Source: CAD feature listing. Evaluate the final solid. Frame: model axes, mm. A direction names the side the tool comes from. Round coordinates to 2 decimals unless told otherwise and drop trailing zeros. Loops run counter-clockwise (first coordinate to the right, second up) from the corner with the lowest first, then second, coordinate; pieces in that order, holes last.
(1) Set-up query: faces 1 (the cylindrical face through (-5.265, -28.594, -3.577)), 2 (the cylindrical face through (-4.88, 43.93, -1.08)), 3 (the flat face through (-22, -58, 0)). Return all of +Z, -Z, +X, -X, +Y, -Y with unobstructed straight access to the full face (end or side cutting, diameter ignored); none if empty.
(2) Material intervals for probe 1 along Y at (x, z) = (0, 2); probe 2 along Y at (x, z) = (0, 9); probe 3 along Z at (x, y) = (-21, -19), sorted ascending.
(3) First-contact query: pin 1 Ø2 at (x, y) = (27, 19) entering from -Z; pin 2 Ø5 at (x, y) = (5, 4) entering from +Z; pin 3 Ø10 at (x, z) = (-13, 28.5) entering from -Y; pin 4 Ø5.5 at (x, y) = (0, 31) entering from +Z. Flat tips, straight axial feed; report the tip coordinate or a pass-through.
(4) Section B-B, the plane z = 0. Return the cut outline in (x, y).
(5) Section D-D, the plane x = -17. Return the cut outline in (y, z), plus the area to 3 significant figures.
(6) Section C-C, the plane y = 31. Return the cut outline in (x, z), plus the area to 3 significant figures.
(7) Section A-A, the plane x = 0. Return the cut outline in (y, z).
(8) Mould query, pull axis Y, two halves, no side actions, for faces 4 (the flat face through (0, 49, 0)), 5 (the cylindrical face through (-2.21, 33.03, 0.53)), 6 (the flat face through (1, 0, -1)). Classes: pulls with the +Y half, pulls with the -Y half, needs draft (parallel to the pull), parting line crosses it, or undercut.
```python
from build123d import *

# Parameters (mm, degrees)
SKETCH_1_R         = 38
EXTRUDE_1_DEPTH    = 39
SKETCH_2_R         = 5
EXTRUDE_2_DEPTH    = 10
SKETCH_6_R         = 16.5
EXTRUDE_6_DEPTH    = 58
SKETCH1_R          = 3
CUT_EXTRUDE1_DEPTH = 50


with BuildPart() as part:
    # Эскиз1 → Вытянуть1 (new body)
    with BuildSketch(Plane(origin=(0, 0, 0), x_dir=(1, 0, 0), z_dir=(0, 1, 0))):
        with Locations(Location((0, 0, 0), (0, 0, 270))):
            Circle(SKETCH_1_R)
    extrude(amount=EXTRUDE_1_DEPTH)

    # Эскиз2 → Вытянуть2 (add)
    with BuildSketch(Plane(origin=(0, 39, 0), x_dir=(1, 0, 0), z_dir=(0, 1, 0))):
        with Locations(Location((0, 0, 0), (0, 0, 270))):
            Circle(SKETCH_2_R)
    extrude(amount=EXTRUDE_2_DEPTH)

    # Эскиз6 → Вытянуть6 (add)
    with BuildSketch(Plane.XZ):
        with Locations(Location((-21.372740523, 0, 0), (0, 0, 90))):
            Circle(SKETCH_6_R)
    extrude(amount=EXTRUDE_6_DEPTH)

    # Sketch1 → Cut-Extrude1 (cut, symmetric)
    with BuildSketch(Plane.XY):
        with Locations((0, 31)):
            Circle(SKETCH1_R)
    extrude(amount=CUT_EXTRUDE1_DEPTH, both=True, mode=Mode.SUBTRACT)


solid = part.part
```
Output values:
1. face 1: -Y
1. face 2: +Y
1. face 3: +Z, -Z, +X, -X, -Y
2. probe 1: y = 0 to 28, 34 to 49
2. probe 2: y = 0 to 28, 34 to 39
2. probe 3: z = -16.5 to 16.5
3. pin 1: stops at z = -27.71
3. pin 2: stops at z = 37.92
3. pin 3: stops at y = 0
3. pin 4: passes through
4. outline: (-38, 0) - (-37.87, 0) - (-37.87, -58) - (-4.87, -58) - (-4.87, 0) - (38, 0) - (38, 39) - (5, 39) - (5, 49) - (-5, 49) - (-5, 39) - (-38, 39) - close; hole circle Ø6 at (0, 31)
5. outline: (-58, -15.91) - (0, -15.91) - (0, -33.99) - (39, -33.99) - (39, 33.99) - (0, 33.99) - (0, 15.91) - (-58, 15.91) - close
5. area: 4,500 mm2
6. outline: (-3, -37.88) - (-3, 37.88) arc R38 ccw to start; (3, -37.88) arc R38 ccw to (3, 37.88) - close
6. area: 4,080 mm2
7. outline: (0, -38) - (28, -38) - (28, 38) - (0, 38) - close; (34, -38) - (39, -38) - (39, -5) - (49, -5) - (49, 5) - (39, 5) - (39, 38) - (34, 38) - close
8. face 4: pulls with the +Y half
8. face 5: undercut
8. face 6: pulls with the -Y half
